Geometry: final body of the model. Coordinates: model frame, mm. A direction names the side the tool comes from. Coordinates: 2 decimals unless noted, no trailing zeros. Order: outer loops, then holes, each group sorted by start corner. A loop starts at its lowest first (then second) coordinate and runs counter-clockwise, first axis right, second up. Notation, with made-up numbers: (8, 10) -> (54, 10) arc R12 cw to (54, 21) -> close; hole circle Ø1 at (89.5, -18). An arc over 180 degrees is marked (long way). Answer in a Markdown table with one row per item. Add a question column.
1) Pull-direction query (Y, two-part tool) for faces 4 (the face through (0, -6.2, -7.5)), 5 (the face through (17, -7.3, -3)), 6 (the face through (9, 0, -7)); classes: +Y half, -Y half, draft (parallel to the pull), parting line (faces both ways), or undercut.
2) Section query D-D on z = -8. Return the cut outline in (x, y), then the cut area to 3 significant figures.
3) Section query C-C on x = 10.25. Return the cut outline in (y, z), then the cut area to 3 significant figures.
4) Set-up query: faces 1 (the face through (3, -7.3, -3)), 2 (the face through (6, -3, -6.3)), 3 (the face through (12, -6, -12.6)). Return all of +Z, -Z, +X, -X, +Y, -Y with unobstructed straight access to the full face (end or side cutting, diameter ignored); none if empty.
5) Ray query, line 1 (Y direction, x = 11, z = -6.3); line 2 (X direction, y = -8.5, z = -4). Return the intervals inside material, ascending. Write a range as from..to.
6) Section query B-B on z = -3. Return the cut outline in (x, y).
7) Contact query for flat-ended pins moving along their axis: P1, Ø8, axis at x = 4, z = -9, coming from the +Y side; P2, Ø1, axis at x = 16.5, y = -11, coming from the -Z side. Output: stop coordinate, or through.
8) Section query A-A on y = -6.3. Return the cut outline in (x, z).
```python
from build123d import *

# Parameters (mm, degrees)
F1_DEPTH  = 12.6
F2_W      = 2
F2_H      = 6.3
F3_DEPTH  = 12.601
F4_W      = 2
F4_H      = 6.2
F5_DEPTH  = 7.2
F6_W      = 3.5
F6_H      = 2
F7_DEPTH  = 12.601
F8_W      = 3.5
F8_H      = 2
F9_DEPTH  = 15.201
F10_R     = 1
F11_DEPTH = 15.401


with BuildPart() as f1:
    # F0 (on Front) → F1 (new body)
    with BuildSketch(Plane.XZ):
        Polygon((18.9, 0), (0, 0), (0, -12.6), (0, -15.2), (4.7, -15.2), (6.2, -12.6), (18.9, -12.6), align=None)
    extrude(amount=F1_DEPTH)

    # F2 (on face) → F3 (cut, through all)
    with BuildSketch(Plane.XZ.offset(12.6)):
        with Locations((6.2, -3.15)):
            Rectangle(F2_W, F2_H)
    extrude(amount=-F3_DEPTH, mode=Mode.SUBTRACT)

    # F4 (on face) → F5 (cut)
    with BuildSketch(Plane(origin=(0, 0, 0), x_dir=(0, -1, 0), z_dir=(-1, 0, 0))):
        with Locations((6.3, -3.1)):
            Rectangle(F4_W, F4_H)
    extrude(amount=-F5_DEPTH, mode=Mode.SUBTRACT)

    # F6 (on face) → F7 (cut, through all)
    with BuildSketch(Plane.XZ.offset(12.6)):
        with Locations((17.15, -6.3)):
            Rectangle(F6_W, F6_H)
    extrude(amount=-F7_DEPTH, mode=Mode.SUBTRACT)

    # F8 (on face) → F9 (cut, through all)
    with BuildSketch(Plane.XY):
        with Locations((17.15, -6.3)):
            Rectangle(F8_W, F8_H)
    extrude(amount=-F9_DEPTH, mode=Mode.SUBTRACT)

    # F10 (on face) → F11 (cut, through all)
    with BuildSketch(Plane.YZ.offset(15.4)):
        with Locations((-6.3, -6.3)):
            Circle(F10_R)
    extrude(amount=-F11_DEPTH, mode=Mode.SUBTRACT)


solid = f1.part
```
Result:
| question | item | result |
|---|---|---|
| 1 | face 4 | draft |
| 1 | face 5 | undercut |
| 1 | face 6 | +Y half |
| 2 | outline | (0, -12.6) -> (18.9, -12.6) -> (18.9, -7.3) -> (15.4, -7.3) -> (15.4, -5.3) -> (18.9, -5.3) -> (18.9, 0) -> (0, 0) -> close |
| 2 | area | 231 mm2 |
| 3 | outline | (-12.6, -12.6) -> (0, -12.6) -> (0, 0) -> (-12.6, 0) -> close; hole circle Ø2 at (-6.3, -6.3) |
| 3 | area | 156 mm2 |
| 4 | face 1 | +Z, -X |
| 4 | face 2 | +Z, +Y, -Y |
| 4 | face 3 | -Z, +X, +Y, -Y |
| 5 | line 1 | -12.6..-7.3, -5.3..0 |
| 5 | line 2 | 0..5.2, 7.2..18.9 |
| 6 | outline | (0, -12.6) -> (5.2, -12.6) -> (5.2, -7.3) -> (0, -7.3) -> close; (0, -5.3) -> (5.2, -5.3) -> (5.2, 0) -> (0, 0) -> close; (7.2, -12.6) -> (18.9, -12.6) -> (18.9, -7.3) -> (15.4, -7.3) -> (15.4, -5.3) -> (18.9, -5.3) -> (18.9, 0) -> (7.2, 0) -> close |
| 7 | P1 | y = 0 |
| 7 | P2 | z = -12.6 |
| 8 | outline | (0, -15.2) -> (4.7, -15.2) -> (6.2, -12.6) -> (15.4, -12.6) -> (15.4, -7.3) -> (0, -7.3) -> close; (7.2, -5.3) -> (15.4, -5.3) -> (15.4, 0) -> (7.2, 0) -> close |
